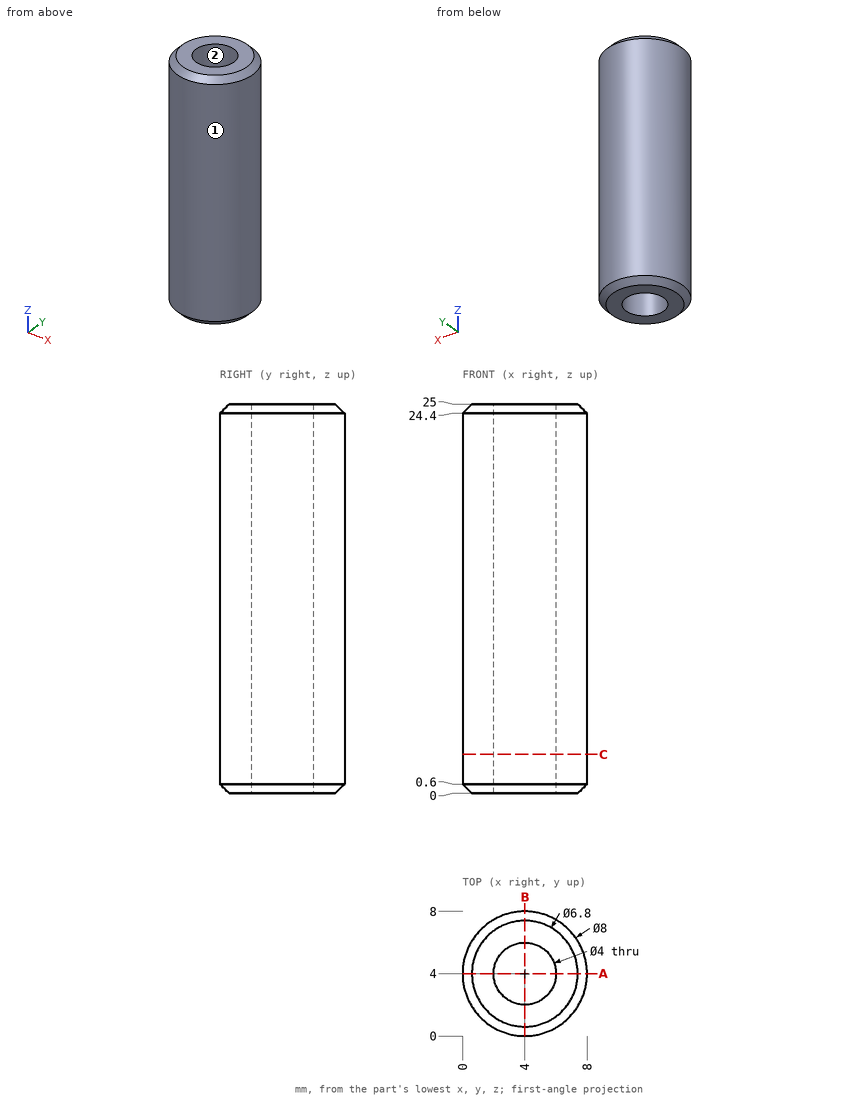
Study the drawing (mm; zero at the part's minimum x, y, z) and answer. Coordinates: 2 decimals unless noted, no trailing zeros. Write each loop counter-clockwise with the first axis right and the second up, starting at its lowest first coordinate (ties: lowest second). Pieces come first, ordered by that corner, then holes. Notation, with made-up numbers: M 9.25,69 L 48.25,69 A18 ccw 48.25,86 Z; hole C -1,27.5 d10. An arc over 180 degrees is marked long. Use one line per item in the form item = value.
Item 1: Find the intervals of material crossed by probe 1 along Y at (x, z) = (4, 9); probe 2 along X at (y, z) = (3, 13.5); probe 3 along Y at (x, z) = (3.5, 13), in increasing order.
Model answer:
probe_1 = 0 to 2, 6 to 8
probe_2 = 0.13 to 2.27, 5.73 to 7.87
probe_3 = 0.03 to 2.06, 5.94 to 7.97
Item 2: Find section C-C, the plane z = 2.5. Give the vertices of the cut face in (x, y).
Model answer:
outline = C 4,4 d8; hole C 4,4 d4
Item 3: The mould has two halves that part along X. Classify the marked faces 1 and 2: released by +X, released by -X, zero draft, split by the parting line, or undercut.
Model answer:
face_1 = split by the parting line
face_2 = undercut
Item 4: Find section A-A, the plane y = 4. Give the vertices of the cut face in (x, z), plus the area to 3 significant figures.
Model answer:
outline = M 0,0.6 L 0.6,0 L 2,0 L 2,25 L 0.6,25 L 0,24.4 Z; M 6,0 L 7.4,0 L 8,0.6 L 8,24.4 L 7.4,25 L 6,25 Z
area = 99.3 mm2
Item 5: Given P1, Ø3, axis at x = 6, z = 9, coming from the -Y side, flat-ended and moving along its own axis, determine where the tip first touches the part or whether it passes through.
Model answer:
P1 = 0.03
